Check sheet for the drawn part. Datum: minimum x, y, z corner. Units: mm. A direction names the side the tool comes from. Coordinates: 2 decimals unless noted, no trailing zeros. Order: outer loops, then holes, each group sorted by start corner. A loop starts at its lowest first (then second) coordinate and runs counter-clockwise, first axis right, second up. Notation, with made-up numbers: (10, 80.25) - (28, 80.25) arc R29 cw to (28, 116.25) - close; hole circle Ø3 at (-20.75, 14.5). An arc over 180 degrees is marked (long way). Put each result on its own line as item: value.
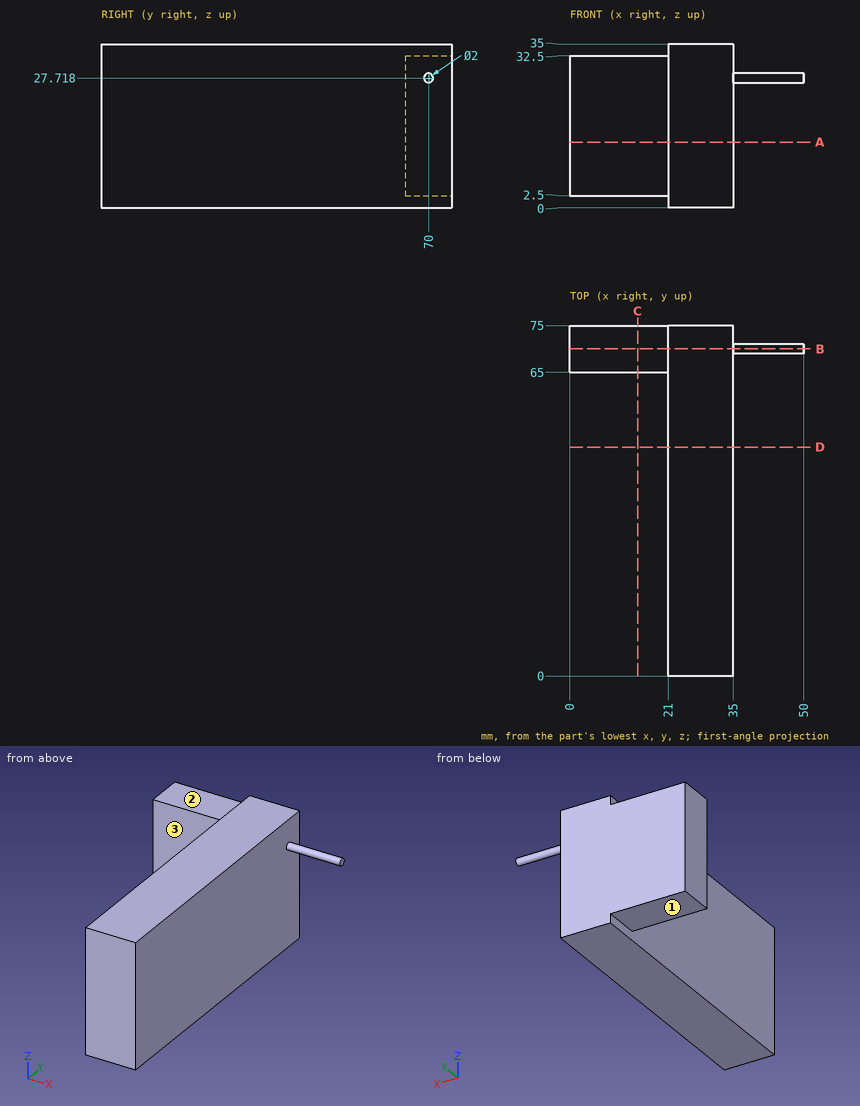
Q1. Section check D-D on y = 49. Record the boundary of the cut face in (x, z).
Answer block:
outline: (21, 0) - (35, 0) - (35, 35) - (21, 35) - close
Q2. Access from +Z, -Z, +X, -X, +Y, -Y to the whole of each face (thin tool, end or side, straight path). Record for the marked faces 1, 2 and 3.
Answer block:
face 1: -Z, -X, +Y, -Y
face 2: +Z, -X, +Y, -Y
face 3: +Z, -Z, -X, -Y
Q3. Section check A-A on z = 14. Record the boundary of the cut face in (x, y), then the cut area to 3 significant figures.
Answer block:
outline: (0, 65) - (21, 65) - (21, 0) - (35, 0) - (35, 75) - (0, 75) - close
area: 1,260 mm^2
Q4. Section check C-C on x = 14.5. Record the boundary of the cut face in (y, z).
Answer block:
outline: (65, 2.5) - (75, 2.5) - (75, 32.5) - (65, 32.5) - close
Q5. Depth check by flat-ended pin: pin 1 Ø17.5 at (y, z) = (19.5, 18) entering from +X; pin 2 Ø11 at (x, y) = (13.5, 69) entering from -Z; pin 3 Ø5 at (y, z) = (15, 23.5) entering from -X. Enter the tip coordinate at first touch or a pass-through.
Answer block:
pin 1: stops at x = 35
pin 2: stops at z = 2.5
pin 3: stops at x = 21
Q6. Section check B-B on y = 70. Record the boundary of the cut face in (x, z), then the cut area to 3 significant figures.
Answer block:
outline: (0, 2.5) - (21, 2.5) - (21, 0) - (35, 0) - (35, 26.72) - (50, 26.72) - (50, 28.72) - (35, 28.72) - (35, 35) - (21, 35) - (21, 32.5) - (0, 32.5) - close
area: 1,150 mm^2
Q7. Thickness scan on L1, parallel to X at y = 33.5, z = 8; L2, parallel to Y at x = 4, z = 18. Record the ranges inside material, lowest first. Write a range as [from, to].
Answer block:
L1: x = [21, 35]
L2: y = [65, 75]
